Check sheet for the modelled part. Datum: model origin and axes. Units: mm. A direction names the side the tool comes from. Give positions to 0.01 mm unless a question says otherwise; leave off trailing zeros. Order: outer loops, then holes, each group sorted by start corner. A loop starts at its lowest first (then second) coordinate and runs counter-clockwise, first axis right, second up. Notation, with made-up numbers: (-8, 86) -> (48, 86) arc R35 cw to (48, 124) -> close; hole circle Ø4 at (44, 73.5). An arc over 180 degrees is marked (long way). One line per question, with ' | ' between items.
```python
from build123d import *

# Parameters (mm, degrees)
BOSS_EXTRUDE1_DEPTH = 40
CUT_EXTRUDE2_DEPTH  = 101.242224803
CUT_EXTRUDE3_DEPTH  = 101.242224803
SKETCH14_R          = 7
CUT_EXTRUDE4_DEPTH  = 101.242224803
CUT_EXTRUDE5_REACH  = 102.242
SKETCH15_R          = 7
SKETCH16_R          = 7
CUT_EXTRUDE6_DEPTH  = 2
CUT_EXTRUDE9_DEPTH  = 6
SKETCH22_W          = 41.976716328
SKETCH22_H          = 31.966333102
CUT_EXTRUDE11_DEPTH = 6
CUT_EXTRUDE12_DEPTH = 6


with BuildPart() as part:
    # Sketch2 → Boss-Extrude1 (new body)
    with BuildSketch(Plane.XY):
        Polygon((60, 58), (71.305705476, 46.694294524), (71.305705476, 11.305705476), (60, 0), (0, 0), (0, 8), (16, 8), (16, 14), (49, 14), (49, 44), (45.974238177, 44), (16, 44), (16, 50), (0, 50), (0, 58), align=None)
    extrude(amount=BOSS_EXTRUDE1_DEPTH)

    # Sketch4 → Cut-Extrude2 (cut, through all)
    with BuildSketch(Plane.XZ):
        with BuildLine():
            Line((0, 25.426887123), (0, 40))
            Line((0, 40), (35.283645911, 40))
            ThreePointArc((35.283645911, 40), (16.196272547, 36.213333337), (0, 25.426887123))
        make_face()
    extrude(amount=-CUT_EXTRUDE2_DEPTH, mode=Mode.SUBTRACT)

    # Sketch12 → Cut-Extrude3 (cut, through all)
    with BuildSketch(Plane(origin=(0, 0, 0), x_dir=(1, 0, 0), z_dir=(0, 1, 0))):
        Polygon((60, 0), (71.305705476, -11.305705476), (71.305705476, 0), align=None)
        Polygon((60, -40), (71.305705476, -28.694294524), (71.305705476, -40), align=None)
    extrude(amount=CUT_EXTRUDE3_DEPTH, mode=Mode.SUBTRACT)

    # Sketch14 → Cut-Extrude4 (cut, through all)
    with BuildSketch(Plane(origin=(71.305705476, 0, 0), x_dir=(0, 0, -1), z_dir=(1, 0, 0))):
        with Locations(Location((-20, 29, 0), (0, 0, 90))):
            Circle(SKETCH14_R)
    extrude(amount=-CUT_EXTRUDE4_DEPTH, mode=Mode.SUBTRACT)

    # Sketch15 → Cut-Extrude5 (cut, up to next)
    with BuildSketch(Plane.XZ, mode=Mode.PRIVATE) as cut_extrude5_sk1:
        with Locations(Location((29, 19, 0), (0, 0, 270))):
            Circle(SKETCH15_R)
    cut_extrude5_tool1 = extrude(cut_extrude5_sk1.sketch, amount=-CUT_EXTRUDE5_REACH, mode=Mode.PRIVATE) & part.part
    add(cut_extrude5_tool1.solids().sort_by_distance((29, 0, 19))[0], mode=Mode.SUBTRACT)

    # Sketch16 → Cut-Extrude6 (cut)
    with BuildSketch(Plane.XZ.offset(-44)):
        with Locations(Location((29, 19, 0), (0, 0, 270))):
            Circle(SKETCH16_R)
    extrude(amount=-CUT_EXTRUDE6_DEPTH, mode=Mode.SUBTRACT)

    # Sketch21 → Cut-Extrude9 (cut)
    with BuildSketch(Plane.XZ):
        with BuildLine():
            Line((0, 22.543268601), (0, 2))
            Line((0, 2), (58, 2))
            Line((58, 2), (58, 38))
            Line((58, 38), (35.283645911, 38))
            ThreePointArc((35.283645911, 38), (16.023283672, 33.966333102), (0, 22.543268601))
        make_face()
    extrude(amount=-CUT_EXTRUDE9_DEPTH, mode=Mode.SUBTRACT)

    # Sketch22 → Cut-Extrude11 (cut)
    with BuildSketch(Plane.XZ.offset(-6)):
        with Locations((37.011641836, 17.983166551)):
            Rectangle(SKETCH22_W, SKETCH22_H)
    extrude(amount=-CUT_EXTRUDE11_DEPTH, mode=Mode.SUBTRACT)

    # Sketch23 → Cut-Extrude12 (cut)
    with BuildSketch(Plane.XZ.offset(-6)):
        with BuildLine():
            Line((16.023283672, 33.966333102), (58, 33.966333102))
            Line((58, 33.966333102), (58, 38))
            Line((58, 38), (34.032069155, 37.983680097))
            ThreePointArc((34.032069155, 37.983680097), (24.80704409, 36.964047425), (16.023283672, 33.966333102))
        make_face()
    extrude(amount=-CUT_EXTRUDE12_DEPTH, mode=Mode.SUBTRACT)


solid = part.part
```
Q1. Section check A-A (y = 29). Enter the section's corners in (x, z), and give its area (3 significant figures).
Result sheet:
outline: (49, 0) -> (60, 0) -> (71.31, 11.31) -> (71.31, 13) -> (49, 13) -> close; (49, 27) -> (71.31, 27) -> (71.31, 28.69) -> (60, 40) -> (49, 40) -> close | area: 452 mm2
Q2. Section check C-C (x = 14). Enter the section's corners in (y, z).
Result sheet:
outline: (0, 0) -> (8, 0) -> (8, 35.24) -> (0, 35.24) -> (0, 33.02) -> (6, 33.02) -> (6, 2) -> (0, 2) -> close; (50, 0) -> (58, 0) -> (58, 35.24) -> (50, 35.24) -> close
Q3. Access from +Z, -Z, +X, -X, +Y, -Y to the whole of each face (thin tool, end or side, straight path). Record for faces 4 (the face through (36, 44, 15)), 5 (the face through (24.93, 8.96, 36.99)), 6 (the face through (16.28, 2.96, 34.08)), 7 (the face through (66, 29, 6)).
Result sheet:
face 4: +Z, -Z, -X | face 5: none | face 6: -Y | face 7: -Z, +X, +Y, -Y
Q4. Thickness scan on line 1 (Y direction, x = 31, z = 32); line 2 (X direction, y = 12.65, z = 19); line 3 (Y direction, x = 14, z = 21). Record the ranges inside material, lowest first.
Result sheet:
line 1: y = 12 to 14, 44 to 58 | line 2: x = 16 to 22, 36 to 71.31 | line 3: y = 6 to 8, 50 to 58
Q5. Depth check by flat-ended pin: pin 1 Ø10 at (x, y) = (7.5, 40) entering from +Z; pin 2 Ø1.8 at (y, z) = (12, 9.5) entering from -X; pin 3 Ø2 at (x, z) = (20, 9) entering from -Y; pin 4 Ø1.8 at (y, z) = (8.5, 22.5) entering from +X. Enter the tip coordinate at first touch or a pass-through.
Result sheet:
pin 1: passes through | pin 2: stops at x = 16 | pin 3: stops at y = 12 | pin 4: stops at x = 69.4
Q6. Mould release check, pull along Y, two halves, no side actions. Record for faces 1 (the face through (24.741, 44.986, 24.555)), 2 (the face through (64, 54, 20)), 3 (the face through (16, 12.3, 17.8)): pulls with the +Y half, pulls with the -Y half, needs draft (parallel to the pull), parting line crosses it, or undercut.
Result sheet:
face 1: needs draft | face 2: pulls with the +Y half | face 3: undercut
Q7. Section check D-D (z = 20). Count the separate pieces of the cut face and the enclosed holes in it, and give its area (3 significant figures).
Result sheet:
separate pieces: 3 | enclosed holes: 0 | area: 1,380 mm2
Q8. Section check B-B (z = 7). Enter the section's corners in (x, y).
Result sheet:
outline: (0, 6) -> (16.02, 6) -> (16.02, 12) -> (58, 12) -> (58, 0) -> (60, 0) -> (67, 7) -> (67, 51) -> (60, 58) -> (0, 58) -> (0, 50) -> (16, 50) -> (16, 44) -> (49, 44) -> (49, 14) -> (16, 14) -> (16, 8) -> (0, 8) -> close
